Geometry: final body of the model. Coordinates: model frame, mm. Face numbers are marked on the shaded views. A direction names the side the tool comes from. Round coordinates to 2 decimals unless told otherwise and drop trailing zeros. Loops run counter-clockwise (first coordinate to the right, second up) from the corner with the lowest first, then second, coordinate; pieces in that order, holes last. Notation, with made-up numbers: M -32,67 L -11,67 A14 cw -11,74 Z; hole C 28,67.25 d10. An arc over 180 degrees is marked long. Answer as a JSON object with one key per item and string values.
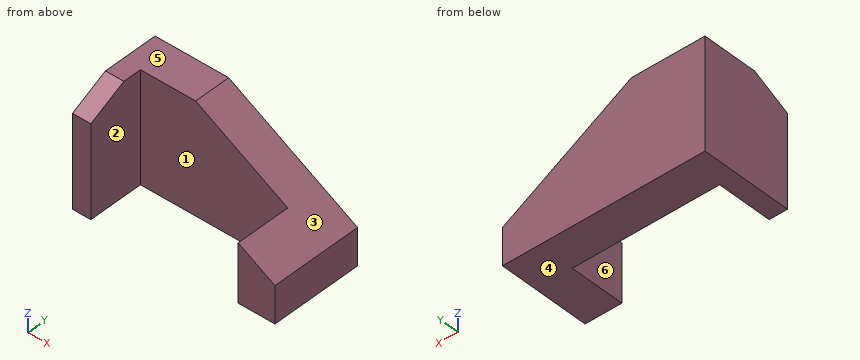
from build123d import *

# Parameters (mm, degrees)
F1_DEPTH = 60
F2_SIZE2 = 10
F2_SIZE  = 20
F3_SIZE2 = 70
F3_SIZE  = 40


with BuildPart() as f1:
    # F0 (on Top) → F1 (new body)
    with BuildSketch(Plane.XY):
        Polygon((0, 50), (0, 0), (10, 0), (10, 30), (90, 30), (90, 0), (110, 0), (110, 50), align=None)
    extrude(amount=F1_DEPTH)

    # F2
    f2_edges = [f1.edges().sort_by_distance(p)[0] for p in [
        (5, 0, 60),
    ]]
    f2_side = f1.faces().sort_by_distance((58.870968, 32.741935, 60))[0]
    chamfer(f2_edges, length=F2_SIZE, length2=F2_SIZE2, reference=f2_side)

    # F3
    f3_edges = [f1.edges().sort_by_distance(p)[0] for p in [
        (110, 25, 60),
    ]]
    f3_side = f1.faces().sort_by_distance((110, 25, 30))[0]
    chamfer(f3_edges, length=F3_SIZE, length2=F3_SIZE2, reference=f3_side)


solid = f1.part
1) Section query C-C (x = 7.5). Return the cut outline in (y, z), and give its area (3 significant figures).
Results:
{"outline": "M 0,0 L 50,0 L 50,60 L 20,60 L 0,50 Z", "area": "2,900 mm2"}
2) Ray query, line 1 (X direction, y = 22, z = 51.5); line 2 (Y direction, x = 83, z = 6); line 3 (Z direction, x = 65, y = 36.5). Return the intervals inside material, ascending.
Results:
{"line 1": "0 to 10", "line 2": "30 to 50", "line 3": "0 to 45.71"}
3) Section query B-B (z = 13). Return the cut outline in (x, y), and give its area (3 significant figures).
Results:
{"outline": "M 0,0 L 10,0 L 10,30 L 90,30 L 90,0 L 110,0 L 110,50 L 0,50 Z", "area": "3,100 mm2"}
4) Pin query (flat end, axial travel): P1, Ø12, axis at x = 78, y = 44.5, coming from the +Z side; P2, Ø6, axis at x = 74.5, z = 40, coming from the -Y side. Return the tip coordinate at first contact, or that it passes through.
Results:
{"P1": "z = 41.71", "P2": "y = 30"}
5) Section query A-A (y = 25.5). Return the cut outline in (x, z), and give its area (3 significant figures).
Results:
{"outline": "M 0,0 L 10,0 L 10,60 L 0,60 Z; M 90,0 L 110,0 L 110,20 L 90,31.43 Z", "area": "1,110 mm2"}
6) Reachability of the marked faces 5 and 6 from +Z, -Z, +X, -X, +Y, -Y: full face, straight path, thin tool, end or side. Return the list, or none.
Results:
{"face 5": "+Z, +X, -X, +Y, -Y", "face 6": "+Z, -Z, -Y"}
7) Section query D-D (y = 13). Return the cut outline in (x, z), and give its area (3 significant figures).
Results:
{"outline": "M 0,0 L 10,0 L 10,56.5 L 0,56.5 Z; M 90,0 L 110,0 L 110,20 L 90,31.43 Z", "area": "1,080 mm2"}
8) Pull-direction query (X, two-part tool) for the marked faces 1, 2, 3 and 4; classes: +X half, -X half, draft (parallel to the pull), parting line (faces both ways), or undercut.
Results:
{"face 1": "undercut", "face 2": "undercut", "face 3": "+X half", "face 4": "draft"}
